from build123d import *

# Parameters (mm, degrees)
F0_R     = 15.24
F1_DEPTH = 25.4


with BuildPart() as f1:
    # F0 (on Top) → F1 (new body)
    with BuildSketch(Plane.XY):
        Polygon((12.519488, 30.841024), (-12.880512, 30.841024), (-30.841024, 12.880512), (-30.841024, -12.519488), (-12.880512, -30.48), (12.519488, -30.48), (30.48, -12.519488), (30.48, 12.880512), align=None)
        Circle(F0_R, mode=Mode.SUBTRACT)
    extrude(amount=F1_DEPTH)


solid = f1.part
Input: part model. Units: mm. Frame: model coordinates. Coordinates: 2 decimals unless noted, no trailing zeros. Loops run counter-clockwise (first coordinate to the right, second up) from the corner with the lowest first, then second, coordinate; pieces in that order, holes last. Notation, with made-up numbers: (58, 59) -> (65, 59) arc R26 cw to (65, 73) -> close; hole circle Ø9 at (-25.75, 52). An arc over 180 degrees is marked (long way). One line per item, written item: value.
(1) Pin query (flat end, axial travel): pin 1 Ø2 at (x, z) = (21.5, 6.5) entering from +Y; pin 2 Ø8 at (y, z) = (19, 3) entering from +X; pin 3 Ø8 at (y, z) = (21, 17) entering from +X. Return the tip coordinate at first contact, or that it passes through.
Answer below:
pin 1: stops at y = 22.86
pin 2: stops at x = 28.36
pin 3: stops at x = 26.36
(2) Ray query, line 1 along Y through (x, z) = (0, 16); line 2 along X through (y, z) = (-12, 8); line 3 along X through (y, z) = (-5, 6). Return the intervals inside material, ascending.
Answer below:
line 1: y = -30.48 to -15.24, 15.24 to 30.84
line 2: x = -30.84 to -9.39, 9.39 to 30.48
line 3: x = -30.84 to -14.4, 14.4 to 30.48
(3) Cut plane D-D (y = -22.5). Output: boundary loops of the cut face in (x, z).
Answer below:
outline: (-20.86, 0) -> (20.5, 0) -> (20.5, 25.4) -> (-20.86, 25.4) -> close
(4) Cut plane A-A (x = 0). Output: boundary loops of the cut face in (y, z).
Answer below:
outline: (-30.48, 0) -> (-15.24, 0) -> (-15.24, 25.4) -> (-30.48, 25.4) -> close; (15.24, 0) -> (30.84, 0) -> (30.84, 25.4) -> (15.24, 25.4) -> close
(5) Draft query along X for faces 1 (the face through (0, -30.48, 13)), 2 (the face through (-3.3, -14.88, 12.52)), 3 (the face through (21.625, 21.735, 12.522)). Return one class per face: pulls with the +X half, pulls with the -X half, needs draft (parallel to the pull), parting line crosses it, or undercut.
Answer below:
face 1: needs draft
face 2: undercut
face 3: pulls with the +X half
(6) Cut plane B-B (z = 2.5). Output: boundary loops of the cut face in (x, y), then the cut area to 3 significant figures.
Answer below:
outline: (-30.84, -12.52) -> (-12.88, -30.48) -> (12.52, -30.48) -> (30.48, -12.52) -> (30.48, 12.88) -> (12.52, 30.84) -> (-12.88, 30.84) -> (-30.84, 12.88) -> close; hole circle Ø30.48 at (0, 0)
area: 2,390 mm2
(7) Cut plane C-C (y = 0). Output: boundary loops of the cut face in (x, z).
Answer below:
outline: (-30.84, 0) -> (-15.24, 0) -> (-15.24, 25.4) -> (-30.84, 25.4) -> close; (15.24, 0) -> (30.48, 0) -> (30.48, 25.4) -> (15.24, 25.4) -> close
